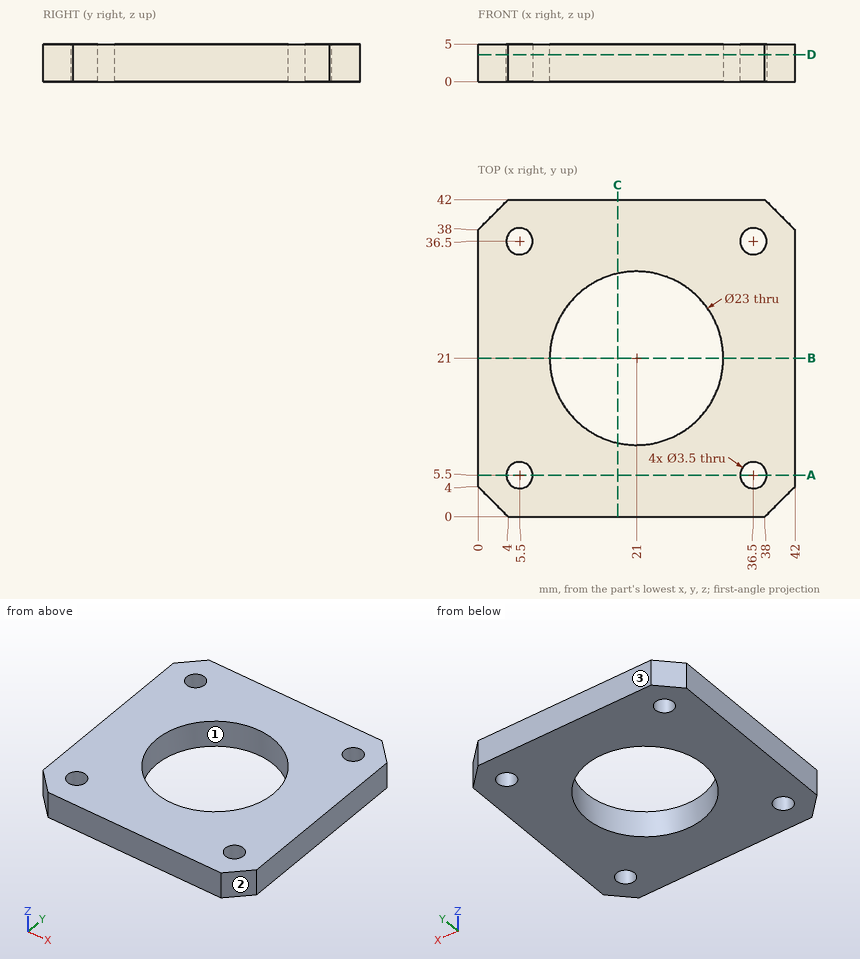
Part print with two shaded views. Sizes in mm from the minimum x, y, z corner. Round coordinates to 2 decimals unless told otherwise and drop trailing zeros. Write each loop counter-clockwise with the first axis right and the second up, starting at its lowest first coordinate (ties: lowest second). Pieces come first, ordered by that corner, then holes. Notation, with made-up numbers: M 23.25,-26 L 82.25,-26 A18 ccw 82.25,2 Z; hole C 55.5,-10 d9. An arc over 180 degrees is marked long. Put each result on its own line as item: value. Start each with the question number.
1) Saw through at C-C, the plane x = 18.5. Write the cut outline in (y, z), and give its area (4 significant figures).
2) Saw through at B-B, the plane y = 21. Write the cut outline in (x, z), and give its area (3 significant figures).
3) Drill centre lines: probe 1 along Y at (x, z) = (5.5, 3.2); probe 2 along Y at (x, z) = (21, 2.95); probe 3 along Y at (x, z) = (4, 2.9). Where is each one in solid material? Low to high. Write a range as [from, to].
4) Saw through at D-D, the plane z = 3.6. Write the cut outline in (x, y), and give its area (3 significant figures).
5) Saw through at A-A, the plane y = 5.5. Write the cut outline in (x, z), and give its area (3 significant figures).
6) Pull direction Y, two halves, no side cores. Call the marked faces 1, 2 and 3: pulls with the +Y half, pulls with the -Y half, needs draft (parallel to the pull), parting line crosses it, or undercut.
Resolved:
1. outline: M 0,0 L 9.78,0 L 9.78,5 L 0,5 Z; M 32.22,0 L 42,0 L 42,5 L 32.22,5 Z
1. area: 97.75 mm²
2. outline: M 0,0 L 9.5,0 L 9.5,5 L 0,5 Z; M 32.5,0 L 42,0 L 42,5 L 32.5,5 Z
2. area: 95.0 mm²
3. probe 1: [0, 3.75], [7.25, 34.75], [38.25, 42]
3. probe 2: [0, 9.5], [32.5, 42]
3. probe 3: [0, 4.6], [6.4, 35.6], [37.4, 42]
4. outline: M 0,4 L 4,0 L 38,0 L 42,4 L 42,38 L 38,42 L 4,42 L 0,38 Z; hole C 5.5,5.5 d3.5; hole C 5.5,36.5 d3.5; hole C 21,21 d23; hole C 36.5,5.5 d3.5; hole C 36.5,36.5 d3.5
4. area: 1,280 mm²
5. outline: M 0,0 L 3.75,0 L 3.75,5 L 0,5 Z; M 7.25,0 L 34.75,0 L 34.75,5 L 7.25,5 Z; M 38.25,0 L 42,0 L 42,5 L 38.25,5 Z
5. area: 175 mm²
6. face 1: undercut
6. face 2: pulls with the -Y half
6. face 3: pulls with the +Y half
